Work out the finished part from the listing and answer in its coordinate system (mm). A direction names the side the tool comes from. Round coordinates to 2 decimals unless told otherwise and drop trailing zeros. Order: outer loops, then holes, each group sorted by start corner. A loop starts at its lowest first (then second) coordinate and runs counter-clockwise, first axis right, second up. Notation, with made-up numbers: (36.5, 4) - (48.5, 4) arc R24 ccw to (48.5, 33) - close; hole circle Ø9 at (-23.75, -19). An arc over 180 degrees is marked (long way). One line per question, with ' | ' between items. Start each with the question number.
from build123d import *

# Parameters (mm, degrees)
F0_R     = 7.493
F1_DEPTH = 9.779


with BuildPart() as f1:
    # F0 (on Top) → F1 (new body)
    with BuildSketch(Plane.XY):
        with BuildLine():
            ThreePointArc((-28.804382, 15.744827), (-39.735006, 11.023195), (-44.236288, 0))
            ThreePointArc((-44.236288, 0), (-39.133073, -11.605518), (-27.130871, -15.689389))
            ThreePointArc((-27.130871, -15.689389), (-26.77073, -15.654057), (-26.411497, -15.610459))
            ThreePointArc((-26.411497, -15.610459), (-13.259182, -13.824655), (0, -13.219206))
            ThreePointArc((0, -13.219206), (13.259182, -13.824655), (26.411497, -15.610459))
            ThreePointArc((26.411497, -15.610459), (44.190629, -1.198327), (28.804382, 15.744827))
            ThreePointArc((28.804382, 15.744827), (28.687684, 15.746024), (28.570993, 15.747783))
            ThreePointArc((28.570993, 15.747783), (20.647303, 17.228065), (13.648412, 21.227016))
            ThreePointArc((13.648412, 21.227016), (11.970991, 22.880077), (10.515754, 24.731734))
            ThreePointArc((10.515754, 24.731734), (0, 30.111899), (-10.515754, 24.731734))
            ThreePointArc((-10.515754, 24.731734), (-11.970991, 22.880077), (-13.648412, 21.227016))
            ThreePointArc((-13.648412, 21.227016), (-20.647303, 17.228065), (-28.570993, 15.747783))
            ThreePointArc((-28.570993, 15.747783), (-28.687684, 15.746024), (-28.804382, 15.744827))
        make_face()
        with BuildLine():
            ThreePointArc((-35.981288, 0), (-28.488288, 7.493), (-20.995288, 0))
            ThreePointArc((-20.995288, 0), (-28.488288, -7.493), (-35.981288, 0))
        make_face(mode=Mode.SUBTRACT)
        with BuildLine():
            ThreePointArc((-14.010288, 0.000393), (-12.397713, 3.848031), (-8.523938, 5.396769))
            Line((-8.523938, 5.396769), (0, 5.389336))
            Line((0, 5.389336), (8.206422, 5.382181))
            ThreePointArc((8.206422, 5.382181), (13.997631, 0.369419), (8.945243, -5.387252))
            Line((8.945243, -5.387252), (-8.945243, -5.387252))
            ThreePointArc((-8.945243, -5.387252), (-12.545316, -3.697057), (-14.010288, 0.000393))
        make_face(mode=Mode.SUBTRACT)
        with Locations((28.488288, 0)):
            Circle(F0_R, mode=Mode.SUBTRACT)
        with BuildLine():
            ThreePointArc((5.3975, 17.14508), (3.816609, 13.328471), (0, 11.74758))
            ThreePointArc((0, 11.74758), (-3.816609, 20.961689), (5.3975, 17.14508))
        make_face(mode=Mode.SUBTRACT)
    extrude(amount=F1_DEPTH)


solid = f1.part
1) For faces 4 (the cylindrical face through (0.17, 30.11, 4.82)), 5 (the cylindrical face through (13.99, 0.49, 4.82)), determine the directions among +Z, -Z, +X, -X, +Y, -Y from which every point of the face is accessible in a straight line to the end or side of a thin tool.
2) Section C-C on y = 20 is taken. Give the vertices of the cut face in (x, z).
3) Flat-ended cylindrical pins translate along their axes: pin 1 (6 mm diameter, centred on x = -29.5, y = 2, fed in from -Z); pin 2 (3 mm diameter, centred on x = 32, z = 5.5, fed in from +Y). Find the tip coordinate at first contact, or state that the pin passes through.
4) Straight lines are drawn through the part: line 1 (Y direction, x = 0.5, z = 1.5); line 2 (X direction, y = 2.5, z = 1.75); line 3 (Y direction, x = -22, z = 8.5). For each, find the intervals that lie inside material, in ascending order.
5) Section B-B on z = 3.75 is taken. Give the number of separate pieces and of enclosed holes in the cut face, and give its area (3 significant figures).
6) Section D-D on x = 19.5 is taken. Give the vertices of the cut face in (y, z), and give its area (3 significant figures).
7) Determine the mould class of faces 1 (the flat face through (0, -5.387, 5)), 2 (the flat face through (-1, 8, 9.779)), 3 (the cylindrical face through (11.99, 22.86, 4.82)) for opening direction Y: released by +Y, released by -Y, zero draft, split by the parting line, or undercut.
8) Section A-A on y = 1.5 is taken. Give the vertices of the cut face in (x, z).
Recorded:
1) face 4: +Z, -Z, +Y | face 5: +Z, -Z
2) outline: (-15.28, 0) - (-4.58, 0) - (-4.58, 9.78) - (-15.28, 9.78) - close; (4.58, 0) - (15.28, 0) - (15.28, 9.78) - (4.58, 9.78) - close
3) pin 1: passes through | pin 2: stops at y = 15.62
4) line 1: y = -13.22 to -5.39, 5.39 to 11.77, 22.52 to 30.1 | line 2: x = -44.04 to -35.55, -21.42 to -13.4, 13.4 to 21.42, 35.55 to 44.04 | line 3: y = -14.88 to -3.75, 3.75 to 16.78
5) separate pieces: 1 | enclosed holes: 4 | area: 2,130 mm²
6) outline: (-14.52, 0) - (17.68, 0) - (17.68, 9.78) - (-14.52, 9.78) - close | area: 315 mm²
7) face 1: undercut | face 2: zero draft | face 3: released by +Y
8) outline: (-44.16, 0) - (-35.83, 0) - (-35.83, 9.78) - (-44.16, 9.78) - close; (-21.15, 0) - (-13.8, 0) - (-13.8, 9.78) - (-21.15, 9.78) - close; (13.8, 0) - (21.15, 0) - (21.15, 9.78) - (13.8, 9.78) - close; (35.83, 0) - (44.16, 0) - (44.16, 9.78) - (35.83, 9.78) - close
